Here's how the part is built. I have some questions about the finished solid (model axes, mm). Round coordinates to 2 decimals unless told otherwise and drop trailing zeros. Loops run counter-clockwise (first coordinate to the right, second up) from the corner with the lowest first, then second, coordinate; pieces in that order, holes last. Notation, with made-up numbers: M 46,72.25 L 66,72.25 A30 ccw 66,95.25 Z; hole C 27,37.25 d7. An arc over 180 degrees is marked long. Answer as a JSON object with one key per item and string values.
from build123d import *

# Parameters (mm, degrees)
PAD_DEPTH    = 3
FILLET_R     = 1
SKETCH002_R  = 3
POCKET_DEPTH = 3.001
FILLET002_R  = 1


with BuildPart() as part:
    # Sketch → Pad (new body)
    with BuildSketch(Plane.XY):
        with BuildLine():
            ThreePointArc((-20, 15), (-35, 0), (-20, -15))
            Line((-20, -15), (20, -15))
            ThreePointArc((20, -15), (35, 0), (20, 15))
            Line((-20, 15), (20, 15))
        make_face()
        with BuildLine():
            ThreePointArc((26.271227, -10.642419), (32, 0), (26.271227, 10.642419))
            ThreePointArc((26.271227, 10.642419), (24.622589, 10.280269), (25.030765, 8.642419))
            ThreePointArc((25.030765, -8.642419), (30, 0), (25.030765, 8.642419))
            ThreePointArc((25.030765, -8.642419), (24.622589, -10.280269), (26.271227, -10.642419))
        make_face(mode=Mode.SUBTRACT)
    extrude(amount=PAD_DEPTH)

    # Fillet
    fillet_edges = [part.edges().sort_by_distance(p)[0] for p in [
        (0, -15, 3),
        (-35, 0, 0),
    ]]
    fillet(fillet_edges, radius=FILLET_R)

    # Sketch002 → Pocket (cut, through all)
    with BuildSketch(Plane(origin=(0, 0, 0), x_dir=(1, 0, 0), z_dir=(0, 0, -1))):
        with Locations((-29, 0)):
            Circle(SKETCH002_R)
    extrude(amount=-POCKET_DEPTH, mode=Mode.SUBTRACT)

    # Fillet002
    fillet002_edges = [part.edges().sort_by_distance(p)[0] for p in [
        (-32, 0, 3),
        (-32, 0, 0),
    ]]
    fillet(fillet002_edges, radius=FILLET002_R)


solid = part.part
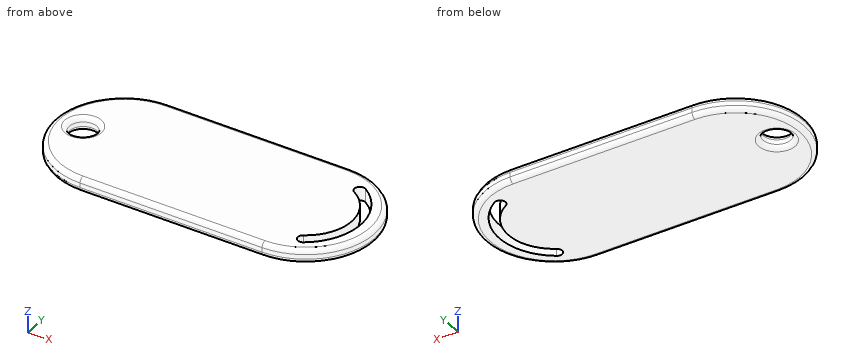
Item 1: I'm going to push flat-ended pins straight in: pin 1 Ø1 at (y, z) = (6.5, 2.5) entering from +X; pin 2 Ø7 at (x, y) = (-29, 0) entering from -Z; pin 3 Ø1 at (x, y) = (-7, 9) entering from -Z. Where does each tip first touch, or does it pass through?
Resolved:
{"pin 1": "x = 33.68", "pin 2": "z = 0.13", "pin 3": "z = 0"}
Item 2: I want a section at A-A, the plane y = 0. Please give me the cut outline in (x, z).
Resolved:
{"outline": "M -35,1 A1 ccw -34,0 L -33,0 A1 ccw -32,1 L -32,2 A1 ccw -33,3 L -34,3 A1 ccw -35,2 Z; M -26,1 A1 ccw -25,0 L 30,0 L 30,3 L -25,3 A1 ccw -26,2 Z; M 32,0 L 34,0 A1 ccw 35,1 L 35,2 A1 ccw 34,3 L 32,3 Z"}
Item 3: Please list where these lines run through material, in increasing order: probe 1 along X at (y, z) = (-8, 0.8); probe 2 along X at (y, z) = (-10.5, 2.45); probe 3 along Y at (x, z) = (-29, 1.45). Write a range as from..to.
Resolved:
{"probe 1": "-32.66..26, 29.18..32.66", "probe 2": "-30.56..24.8, 26.48..30.56", "probe 3": "-12..-3, 3..12"}
Item 4: I want a section at B-B, the plane z = 1.5. Please give me the cut outline in (x, y), then the cut area to 3 significant figures.
Resolved:
{"outline": "M -20,-15 L 20,-15 A15 ccw 20,15 L -20,15 A15 ccw Z; hole C -29,0 d6; hole M 25.03,-8.64 A1.18 ccw long 26.27,-10.64 A12.75 ccw 26.27,10.64 A1.18 ccw long 25.03,8.64 A10 cw Z", "area": "1,830 mm²"}
